Can you work these out from the model? Positions are in its coordinate system, mm. A direction names the side the tool comes from. Round coordinates to 2 decimals unless told otherwise and drop trailing zeros. Write each loop counter-clockwise with the first axis right and the second up, starting at its lowest first coordinate (ties: lowest second). Pieces come first, ordered by that corner, then holes. Notation, with made-up numbers: M 62.25,71.5 L 116.25,71.5 A26 cw 116.25,88.5 Z; hole C 83.25,16.5 d6. An arc over 180 degrees is marked long. Answer as a JSON object with one key per item and string values. Group by question number.
1) Suppose I cut it at B-B, the plane x = 52. Write out the boundary of the cut face in (y, z), and give its area (3 significant figures).
2) If we mould it in two halves opening along X, with no side actions, what happens to faces 4 (the flat face through (0, -1, 46)), 5 (the cylindrical face through (18, 0, 0)), 6 (the flat face through (40, -5, 0))? For each: +X half, -X half, draft (parallel to the pull), parting line (faces both ways), or undercut.
3) Please list where these lines run through material, in increasing order: L1, parallel to X at y = 42, z = 26; L2, parallel to Z at x = 7.5, y = -20.5; L3, parallel to Y at x = 6, z = 22.5. Write a range as [from, to].
4) On a 3-axis mill with a long thin cutter (end or side, diameter ignored), from which of +Z, -Z, +X, -X, +Y, -Y can I reach the whole of each face in a straight line? I mean faces 1 (the cylindrical face through (31.67, 0.81, 44.99)), 2 (the flat face through (39, -60, 0)), 3 (the flat face through (35, 40, 29)). Say none if no direction works.
5) Suppose I cut it at A-A, the plane y = 0. Write out the boundary of the cut face in (x, z).
6) I'm going to push flat-ended pins straight in: pin 1 Ø2 at (x, z) = (9, 26) entering from +Y; pin 2 Ø1.5 at (x, z) = (55, 25.5) entering from +Y; pin 3 Ø5 at (x, z) = (38, 16.5) entering from -Y. Where does each tip first touch, or does it pass through?
7) Suppose I cut it at D-D, the plane y = 38. Write out the boundary of the cut face in (x, z).
8) Suppose I cut it at C-C, the plane z = 34. Write out the boundary of the cut face in (x, y).
from build123d import *

# Parameters (mm, degrees)
F0_W     = 120
F0_H     = 10
F1_DEPTH = 80
F3_DEPTH = 80.001
F4_DEPTH = 25
F5_W     = 10
F5_H     = 10
F6_DEPTH = 70.001


with BuildPart() as f1:
    # F0 (on Right) → F1 (new body)
    with BuildSketch(Plane.YZ):
        Rectangle(F0_W, F0_H)
        with BuildLine():
            ThreePointArc((60, 5), (0, 65), (-60, 5))
            Line((-60, 5), (60, 5))
        make_face()
    extrude(amount=F1_DEPTH)

    # F2 (on face) → F3 (cut, through all)
    with BuildSketch(Plane.YZ.offset(80)):
        with BuildLine():
            Line((-5, 5), (5, 5))
            ThreePointArc((5, 5), (0, 10), (-5, 5))
        make_face()
        with BuildLine():
            ThreePointArc((-5, 5), (0, 0), (5, 5))
            Line((5, 5), (-5, 5))
        make_face()
        with BuildLine():
            ThreePointArc((-5, 5), (0, 10), (5, 5))
            Line((5, 5), (35, 5))
            ThreePointArc((35, 5), (36.3556550657, 8.4232659844), (39.6875, 9.9902248196))
            ThreePointArc((39.6875, 9.9902248196), (0, 45), (-39.6875, 9.9902248196))
            ThreePointArc((-39.6875, 9.9902248196), (-36.3556550657, 8.4232659844), (-35, 5))
            Line((-35, 5), (-5, 5))
        make_face()
        with BuildLine():
            Line((40, 5), (35, 5))
            ThreePointArc((35, 5), (40, 0), (45, 5))
            ThreePointArc((45, 5), (43.4232659844, 8.6443449343), (39.6875, 9.9902248196))
            ThreePointArc((39.6875, 9.9902248196), (39.9217985567, 7.5), (40, 5))
        make_face()
        with BuildLine():
            ThreePointArc((39.6875, 9.9902248196), (36.3556550657, 8.4232659844), (35, 5))
            Line((35, 5), (40, 5))
            ThreePointArc((40, 5), (39.9217985567, 7.5), (39.6875, 9.9902248196))
        make_face()
        with BuildLine():
            Line((-40, 5), (-35, 5))
            ThreePointArc((-35, 5), (-36.3556550657, 8.4232659844), (-39.6875, 9.9902248196))
            ThreePointArc((-39.6875, 9.9902248196), (-39.9217985567, 7.5), (-40, 5))
        make_face()
        with BuildLine():
            ThreePointArc((-39.6875, 9.9902248196), (-43.6443449343, 1.5767340156), (-35, 5))
            Line((-35, 5), (-40, 5))
            ThreePointArc((-40, 5), (-39.9217985567, 7.5), (-39.6875, 9.9902248196))
        make_face()
    extrude(amount=-F3_DEPTH, mode=Mode.SUBTRACT)

    # F2 (on face) → F4 (cut)
    with BuildSketch(Plane.YZ.offset(80)):
        with BuildLine():
            Line((-5, 5), (5, 5))
            ThreePointArc((5, 5), (0, 10), (-5, 5))
        make_face()
        with BuildLine():
            ThreePointArc((-5, 5), (0, 0), (5, 5))
            Line((5, 5), (-5, 5))
        make_face()
        with BuildLine():
            ThreePointArc((-5, 5), (0, 10), (5, 5))
            Line((5, 5), (35, 5))
            ThreePointArc((35, 5), (36.3556550657, 8.4232659844), (39.6875, 9.9902248196))
            ThreePointArc((39.6875, 9.9902248196), (0, 45), (-39.6875, 9.9902248196))
            ThreePointArc((-39.6875, 9.9902248196), (-36.3556550657, 8.4232659844), (-35, 5))
            Line((-35, 5), (-5, 5))
        make_face()
        with BuildLine():
            Line((40, 5), (35, 5))
            ThreePointArc((35, 5), (40, 0), (45, 5))
            ThreePointArc((45, 5), (43.4232659844, 8.6443449343), (39.6875, 9.9902248196))
            ThreePointArc((39.6875, 9.9902248196), (39.9217985567, 7.5), (40, 5))
        make_face()
        with BuildLine():
            ThreePointArc((39.6875, 9.9902248196), (36.3556550657, 8.4232659844), (35, 5))
            Line((35, 5), (40, 5))
            ThreePointArc((40, 5), (39.9217985567, 7.5), (39.6875, 9.9902248196))
        make_face()
        with BuildLine():
            Line((-40, 5), (-35, 5))
            ThreePointArc((-35, 5), (-36.3556550657, 8.4232659844), (-39.6875, 9.9902248196))
            ThreePointArc((-39.6875, 9.9902248196), (-39.9217985567, 7.5), (-40, 5))
        make_face()
        with BuildLine():
            ThreePointArc((-39.6875, 9.9902248196), (-43.6443449343, 1.5767340156), (-35, 5))
            Line((-35, 5), (-40, 5))
            ThreePointArc((-40, 5), (-39.9217985567, 7.5), (-39.6875, 9.9902248196))
        make_face()
    extrude(amount=-F4_DEPTH, mode=Mode.SUBTRACT)

    # F5 (on face) → F6 (cut, through all)
    with BuildSketch(Plane(origin=(0, 0, -5), x_dir=(1, 0, 0), z_dir=(0, 0, -1))):
        with Locations((40, 40)):
            Rectangle(F5_W, F5_H)
        with Locations((40, 0)):
            Rectangle(F5_W, F5_H)
        with Locations((40, -40)):
            Rectangle(F5_W, F5_H)
    extrude(amount=-F6_DEPTH, mode=Mode.SUBTRACT)


solid = f1.part
Results:
{
 "1": {"outline": "M -60,-5 L 60,-5 L 60,5 A60 ccw -60,5 Z; hole M -39.69,9.99 A5 ccw long -35,5 L -5,5 A5 ccw 5,5 L 35,5 A5 ccw long 39.69,9.99 A40 ccw Z", "area": "4,180 mm^2"},
 "2": {"face 4": "-X half", "face 5": "draft", "face 6": "undercut"},
 "3": {"L1": "[0, 35], [45, 80]", "L2": "[-5, 5], [39.35, 61.39]", "L3": "[-57.39, -35.97], [35.97, 57.39]"},
 "4": {"face 1": "+X, -X", "face 2": "+Z, -Z, +X, -X, -Y", "face 3": "+Z, -Z"},
 "5": {"outline": "M 0,-5 L 35,-5 L 35,0 L 0,0 Z; M 0,45 L 35,45 L 35,65 L 0,65 Z; M 45,-5 L 80,-5 L 80,0 L 45,0 Z; M 45,45 L 80,45 L 80,65 L 45,65 Z"},
 "6": {"pin 1": "y = 56.57", "pin 2": "y = 56.66", "pin 3": "y = -59.32"},
 "7": {"outline": "M 0,-5 L 35,-5 L 35,0.42 L 0,0.42 Z; M 0,17.49 L 35,17.49 L 35,51.43 L 0,51.43 Z; M 45,-5 L 80,-5 L 80,0.42 L 45,0.42 Z; M 45,17.49 L 80,17.49 L 80,51.43 L 45,51.43 Z"},
 "8": {"outline": "M 0,-52.53 L 80,-52.53 L 80,-27.55 L 0,-27.55 Z; M 0,27.55 L 80,27.55 L 80,52.53 L 0,52.53 Z; hole M 35,-45 L 45,-45 L 45,-35 L 35,-35 Z; hole M 35,35 L 45,35 L 45,45 L 35,45 Z"}
}
